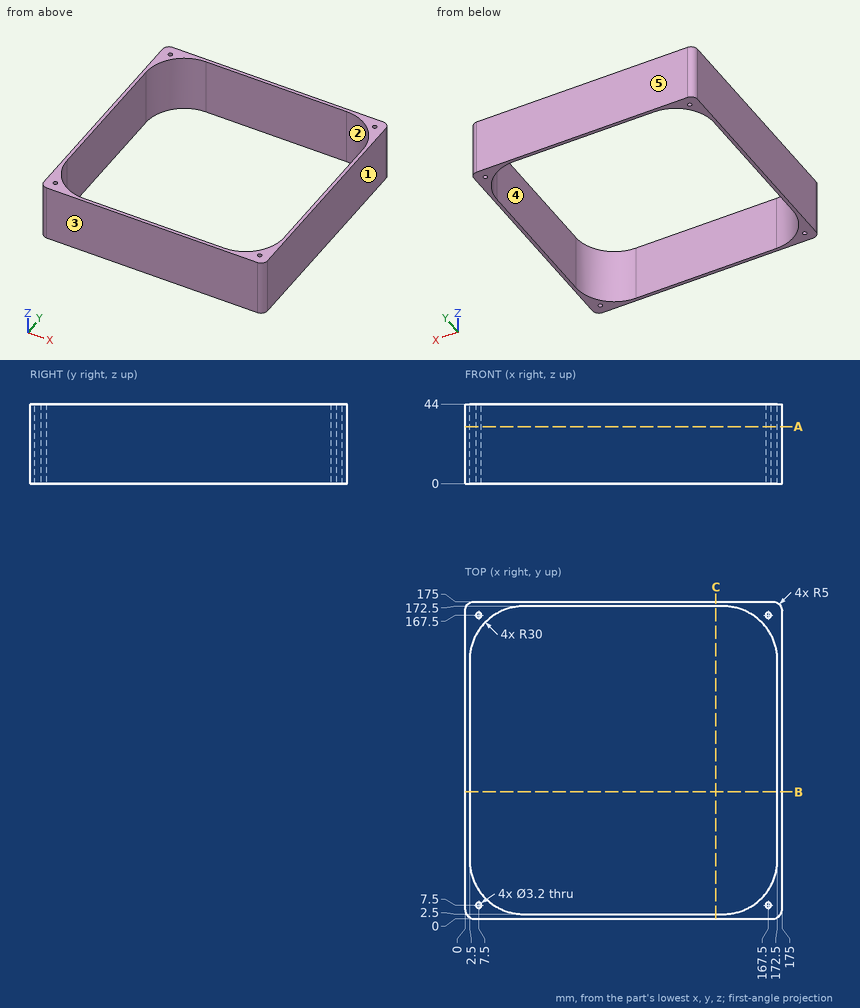
Here's the drawing with two shaded views (mm, measured from the low corner). I have some questions. A direction names the side the tool comes from. Round coordinates to 2 decimals unless told otherwise and drop trailing zeros. Order: outer loops, then holes, each group sorted by start corner. A loop starts at its lowest first (then second) coordinate and runs counter-clockwise, first axis right, second up. Notation, with made-up numbers: M -24.75,-0.75 L 3.25,-0.75 A6 ccw 3.25,4.25 Z; hole C -21,-33.5 d7. An arc over 180 degrees is marked long. Use CSV: the item, a comma, the result in double quotes.
1) I want a section at B-B (y = 70). List the corners of the cut face in (x, z) for me, then the cut area to 3 significant figures.
Taken from the geometry:
outline,"M 0,0 L 2.5,0 L 2.5,44 L 0,44 Z; M 172.5,0 L 175,0 L 175,44 L 172.5,44 Z"
area,"220 mm^2"
2) I'm going to push a flat-ended pin straight in: P1, Ø1.9, axis at x = 167.5, y = 7.5, coming from the +Z side. Where does the tip first touch, or does it pass through?
Taken from the geometry:
P1,"through"
3) If we mould it in two halves opening along X, with no side actions, what happens to the marked faces 1, 2 and 3? For each: pulls with the +X half, pulls with the -X half, needs draft (parallel to the pull), parting line crosses it, or undercut.
Taken from the geometry:
face 1,"pulls with the +X half"
face 2,"undercut"
face 3,"needs draft"
4) I need wall thicknesses on line 1 along X through (y, z) = (141.5, 6); line 2 along Y through (x, z) = (167.5, 23.5); line 3 along X through (y, z) = (167, 33). Which ranges of each line are inside material? Lowest first, please. Write a range as [from, to].
Taken from the geometry:
line 1,"[0, 2.5], [172.5, 175]"
line 2,"[0, 5.9], [9.1, 15.92], [159.08, 165.9], [169.1, 175]"
line 3,"[0, 5.98], [9.02, 15.19], [159.81, 165.98], [169.02, 175]"
5) On a 3-axis mill with a long thin cutter (end or side, diameter ignored), from which of +Z, -Z, +X, -X, +Y, -Y can I reach the whole of each face in a straight line? I mean the marked faces 4 and 5. Say none if no direction works.
Taken from the geometry:
face 4,"+Z, -Z"
face 5,"+Z, -Z, +X, -X, +Y"
6) I want a section at A-A (z = 31.5). List the corners of the cut face in (x, y) for me.
Taken from the geometry:
outline,"M 0,5 A5 ccw 5,0 L 170,0 A5 ccw 175,5 L 175,170 A5 ccw 170,175 L 5,175 A5 ccw 0,170 Z; hole M 2.5,32.5 A30 ccw 32.5,2.5 L 142.5,2.5 A30 ccw 172.5,32.5 L 172.5,142.5 A30 ccw 142.5,172.5 L 32.5,172.5 A30 ccw 2.5,142.5 Z; hole C 7.5,7.5 d3.2; hole C 7.5,167.5 d3.2; hole C 167.5,7.5 d3.2; hole C 167.5,167.5 d3.2"
